from build123d import *

# Parameters (mm, degrees)
SKETCH1_W                                       = 152.4
SKETCH1_H                                       = 177.8
BOSS_EXTRUDE1_DEPTH                             = 12.7
SKETCH3_R                                       = 25.4
CUT_EXTRUDE2_DEPTH                              = 118.774954893
CBORE_FOR_10_SOCKET_HEAD_CAP_SCREW2_D           = 5.1054
CBORE_FOR_10_SOCKET_HEAD_CAP_SCREW2_CBORE_D     = 9.525
CBORE_FOR_10_SOCKET_HEAD_CAP_SCREW2_CBORE_DEPTH = 4.826
MIRROR5_COPY_1_D                                = 5.1054
MIRROR5_COPY_1_CBORE_D                          = 9.525
MIRROR5_COPY_1_CBORE_DEPTH                      = 4.826
SKETCH21_W                                      = 177.8
SKETCH21_H                                      = 19.05
CUT_EXTRUDE7_DEPTH                              = 1.27
SKETCH22_R                                      = 6.604
CUT_EXTRUDE8_DEPTH                              = 8.89
CIRPATTERN4_COUNT                               = 4
CIRPATTERN5_COUNT                               = 4
CHAMFER1_SIZE                                   = 7.62
CUT_EXTRUDE15_DEPTH                             = 2.032


with BuildPart() as part:
    # Sketch1 → Boss-Extrude1 (new body)
    with BuildSketch(Plane.XY):
        Rectangle(SKETCH1_W, SKETCH1_H)
    extrude(amount=BOSS_EXTRUDE1_DEPTH)

    # Sketch3 → Cut-Extrude2 (cut, through all)
    with BuildSketch(Plane(origin=(0, 0, 0), x_dir=(-1, 0, 0), z_dir=(0, 0, -1))):
        Circle(SKETCH3_R)
    extrude(amount=-CUT_EXTRUDE2_DEPTH, mode=Mode.SUBTRACT)

    # CBORE for #10 Socket Head Cap Screw2 (through all)
    with Locations(Plane.XY.offset(12.7)):
        with Locations((71.12, 72.009), (0, 72.009), (71.12, 0)):
            cbore_for_10_socket_head_cap_screw2 = CounterBoreHole(CBORE_FOR_10_SOCKET_HEAD_CAP_SCREW2_D / 2, CBORE_FOR_10_SOCKET_HEAD_CAP_SCREW2_CBORE_D / 2, CBORE_FOR_10_SOCKET_HEAD_CAP_SCREW2_CBORE_DEPTH)

    # Mirror4: CBORE for #10 Socket Head Cap Screw2 across plane
    add(cbore_for_10_socket_head_cap_screw2.mirror(Plane.ZX), mode=Mode.SUBTRACT)

    # Mirror5: CBORE for #10 Socket Head Cap Screw2 across plane
    add(cbore_for_10_socket_head_cap_screw2.mirror(Plane(origin=(0, 0, 0), x_dir=(0, 0, 1), z_dir=(1, 0, 0))), mode=Mode.SUBTRACT)

    # Mirror5 copy 1 (through all)
    with Locations(Plane(origin=(0, 0, 12.7), x_dir=(-1, 0, 0), z_dir=(0, 0, 1))):
        with Locations((71.12, 72.009), (0, 72.009), (71.12, 0)):
            CounterBoreHole(MIRROR5_COPY_1_D / 2, MIRROR5_COPY_1_CBORE_D / 2, MIRROR5_COPY_1_CBORE_DEPTH)

    # Sketch21 → Cut-Extrude7 (cut)
    with BuildSketch(Plane(origin=(0, 0, 0), x_dir=(-1, 0, 0), z_dir=(0, 0, -1))):
        with Locations((0, 85.471)):
            Rectangle(SKETCH21_W, SKETCH21_H)
    cut_extrude7 = extrude(amount=-CUT_EXTRUDE7_DEPTH, mode=Mode.SUBTRACT)

    # Mirror8: Cut-Extrude7 across plane
    add(cut_extrude7.mirror(Plane.ZX), mode=Mode.SUBTRACT)

    # Sketch22 → Cut-Extrude8 (cut)
    with BuildSketch(Plane(origin=(0, 0, 0), x_dir=(-1, 0, 0), z_dir=(0, 0, -1))):
        with Locations((31.75, 31.75)):
            Circle(SKETCH22_R)
    cut_extrude8 = extrude(amount=-CUT_EXTRUDE8_DEPTH, mode=Mode.SUBTRACT)

    # CirPattern4: Cut-Extrude8 ×4 about axis
    cirpattern4_axis = Axis((0, 0, 0), (0, 0, 1))
    for i in range(1, CIRPATTERN4_COUNT):
        add(cut_extrude8.rotate(cirpattern4_axis, i * 360 / CIRPATTERN4_COUNT), mode=Mode.SUBTRACT)

    # Sketch24 → #6-32 Tapped Hole1 (revolve, cut)
    with BuildSketch(Plane(origin=(0, 28.575, 12.7), x_dir=(0, -1, 0), z_dir=(1, 0, 0))):
        Polygon((0, 0), (0, 5.89269403), (1.35255, 5.08), (1.35255, 0), align=None)
    f_6_32_tapped_hole1 = revolve(axis=Axis((0, 28.575, 19.05), (0, 0, -1)), mode=Mode.SUBTRACT)

    # CirPattern5: #6-32 Tapped Hole1 ×4 about axis
    cirpattern5_axis = Axis((0, 0, 0), (0, 0, 1))
    for i in range(1, CIRPATTERN5_COUNT):
        add(f_6_32_tapped_hole1.rotate(cirpattern5_axis, i * 360 / CIRPATTERN5_COUNT), mode=Mode.SUBTRACT)

    # Chamfer1
    chamfer1_edges = [part.edges().sort_by_distance(p)[0] for p in [
        (25.4, 0, 0),
    ]]
    chamfer(chamfer1_edges, length=CHAMFER1_SIZE)

    # Sketch28 → Cut-Extrude15 (cut)
    with BuildSketch(Plane.XY):
        with BuildLine():
            Line((-62.7507, 67.6275), (62.7507, 67.6275))
            ThreePointArc((62.7507, 67.6275), (66.19911835, 66.19911835), (67.6275, 62.7507))
            Line((67.6275, 62.7507), (67.6275, -62.7507))
            ThreePointArc((67.6275, -62.7507), (66.19911835, -66.19911835), (62.7507, -67.6275))
            Line((62.7507, -67.6275), (-62.7507, -67.6275))
            ThreePointArc((-62.7507, -67.6275), (-66.19911835, -66.19911835), (-67.6275, -62.7507))
            Line((-67.6275, -62.7507), (-67.6275, 62.7507))
            ThreePointArc((-67.6275, 62.7507), (-66.19911835, 66.19911835), (-62.7507, 67.6275))
        make_face()
        with BuildLine():
            Line((-62.7507, 65.2907), (62.7507, 65.2907))
            ThreePointArc((62.7507, 65.2907), (64.546751224, 64.546751224), (65.2907, 62.7507))
            Line((65.2907, 62.7507), (65.2907, -62.7507))
            ThreePointArc((65.2907, -62.7507), (64.546751224, -64.546751224), (62.7507, -65.2907))
            Line((62.7507, -65.2907), (-62.7507, -65.2907))
            ThreePointArc((-62.7507, -65.2907), (-64.546751224, -64.546751224), (-65.2907, -62.7507))
            Line((-65.2907, -62.7507), (-65.2907, 62.7507))
            ThreePointArc((-65.2907, 62.7507), (-64.546751224, 64.546751224), (-62.7507, 65.2907))
        make_face(mode=Mode.SUBTRACT)
    extrude(amount=CUT_EXTRUDE15_DEPTH, mode=Mode.SUBTRACT)


solid = part.part
Read the model definition and answer for the solid it produces. Units are mm, in the model's axes. A direction names the side the tool comes from. Coordinates: 2 decimals unless noted, no trailing zeros. Use a Markdown table: item, result.
Q1. Determine the mould class of faces 4 (the face through (-18, 21, 12.7)), 5 (the face through (68.762, -0.978, 3.882)) for opening direction X: released by +X, released by -X, zero draft, split by the parting line, or undercut.
Answer block:
| item | result |
|---|---|
| face 4 | zero draft |
| face 5 | undercut |
Q2. Which of the six approach directions +Z, -Z, +X, -X, +Y, -Y give full straight-line access (tool end or side, diameter ignored) to faces 1 (the face through (-67.34, -69.11, 10.32)), 2 (the face through (32, -32, 8.89)), 3 (the face through (1, -83, 1.27))?
Answer block:
| item | result |
|---|---|
| face 1 | +Z |
| face 2 | -Z |
| face 3 | -Z, +X, -X, -Y |
Q3. The part is cut by section A-A, the plane x = -71.12. Give the number of separate pieces and of enclosed holes in the cut face, then the cut area to 3 significant figures.
Answer block:
| item | result |
|---|---|
| separate pieces | 4 |
| enclosed holes | 0 |
| area | 1,970 mm2 |
Q4. Each of these flat-tipped pins is pushed along its axis until it touches: pin 1 Ø3 at (x, y) = (-72.5, -73) entering from +Z; pin 2 Ø5 at (x, y) = (25, 66) entering from -Z; pin 3 Ø1 at (x, z) = (21, 0.5) entering from +Y; pin 4 Ø1 at (x, z) = (3.5, 0.5) entering from -Y. Where does it stop, or does it pass through?
Answer block:
| item | result |
|---|---|
| pin 1 | stops at z = 7.87 |
| pin 2 | stops at z = 0 |
| pin 3 | stops at y = 75.95 |
| pin 4 | stops at y = -75.95 |
Q5. Straight lines are drawn through the part: L1, parallel to X at y = -31.75, z = 4.75; L2, parallel to Y at x = -71.12, z = 5; L3, parallel to Y at x = 1, z = 2. For each, find the intervals that lie inside material, in ascending order. Write a range as [from, to].
Answer block:
| item | result |
|---|---|
| L1 | x = [-76.2, -38.35], [-25.15, 25.15], [38.35, 76.2] |
| L2 | y = [-88.9, -74.56], [-69.46, -2.55], [2.55, 69.46], [74.56, 88.9] |
| L3 | y = [-88.9, -74.36], [-69.66, -67.63], [-65.29, -31], [31, 65.29], [67.63, 69.66], [74.36, 88.9] |
